Autodesk Inventor part; units mm, degrees
ref_plane "YZ Plane" through (0, 0, 0) normal (1, 0, 0) x (0, 1, 0)
ref_plane "XZ Plane" through (0, 0, 0) normal (0, 1, 0) x (-1, 0, 0)
ref_plane "XY Plane" through (0, 0, 0) normal (0, 0, 1) x (1, 0, 0)
sketch "Sketch1" plane through (0, 0, 0) normal (0, 0, 1) x (1, 0, 0)
  circle A0 centre (8.7376, -2.3876) radius 2.032
  circle A1 centre (-8.7376, -2.3876) radius 2.032
  arc A2 (9.5508, 6.3501) -> (10.564, 6.3532) centre (10.0574, 6.3501) ccw
  line L0 (9.5508, 6.3501) -> (6.3306, 6.3501)
  arc A3 (5.3174, 6.3501) -> (6.3306, 6.3501) centre (5.824, 6.3501) ccw
  line L1 (5.3174, 6.3501) -> (4.2872, 6.3501)
  arc A4 (4.2872, 6.3501) -> (3.2382, 5.3011) centre (4.2872, 5.3011) ccw
  line L2 (3.2382, 5.3011) -> (3.2382, 5.1893)
  arc A5 (3.2382, 5.1893) -> (4.2872, 4.1403) centre (4.2872, 5.1893) ccw
  line L3 (4.2872, 4.1403) -> (6.5409, 4.1403)
  arc A6 (7.2003, 2.5463) -> (6.5409, 4.1403) centre (6.5409, 3.2069) ccw
  line L4 (7.2003, 2.5463) -> (3.8742, -0.7738)
  arc A7 (1.6311, -1.7017) -> (3.8742, -0.7738) centre (1.6311, 1.4733) ccw
  line L5 (1.6311, -1.7017) -> (-1.6318, -1.7017)
  arc A8 (-3.8748, -0.7738) -> (-1.6318, -1.7017) centre (-1.6318, 1.4733) ccw
  line L6 (-3.8748, -0.7738) -> (-7.092, 2.4374)
  arc A9 (-6.3875, 4.1403) -> (-7.092, 2.4374) centre (-6.3875, 3.1432) ccw
  line L7 (-6.3875, 4.1403) -> (-4.2879, 4.1403)
  arc A10 (-4.2879, 4.1403) -> (-3.2388, 5.1893) centre (-4.2879, 5.1893) ccw
  line L8 (-3.2388, 5.1893) -> (-3.2388, 5.3011)
  arc A11 (-3.2388, 5.3011) -> (-4.2879, 6.3501) centre (-4.2879, 5.3011) ccw
  line L9 (-4.2879, 6.3501) -> (-5.3196, 6.3501)
  arc A12 (-6.3328, 6.3501) -> (-5.3196, 6.3501) centre (-5.8262, 6.3501) ccw
  line L10 (-6.3328, 6.3501) -> (-9.5528, 6.3501)
  arc A13 (-10.566, 6.3457) -> (-9.5528, 6.3501) centre (-10.0594, 6.3501) ccw
  line L11 (-10.566, 6.3457) -> (-10.5916, 6.3457)
  arc A14 (-10.5916, 6.3457) -> (-12.7, 4.2373) centre (-10.5916, 4.2373) ccw
  line L12 (-12.7, 4.2373) -> (-12.7, -4.2331)
  arc A15 (-12.7, -4.2331) -> (-10.5647, -6.3413) centre (-10.5916, -4.2331) ccw
  arc A16 (-9.5516, -6.35) -> (-10.5647, -6.3413) centre (-10.0581, -6.3412) ccw
  line L13 (-9.5516, -6.35) -> (-6.323, -6.35)
  arc A17 (-5.31, -6.35) -> (-6.323, -6.35) centre (-5.8165, -6.3412) ccw
  line L14 (-5.31, -6.35) -> (5.31, -6.35)
  arc A18 (6.323, -6.35) -> (5.31, -6.35) centre (5.8165, -6.3412) ccw
  line L15 (6.323, -6.35) -> (9.5502, -6.35)
  arc A19 (10.5633, -6.3403) -> (9.5502, -6.35) centre (10.0567, -6.3412) ccw
  line L16 (10.5633, -6.3403) -> (10.589, -6.3404)
  arc A20 (10.589, -6.3404) -> (12.6991, -4.2321) centre (10.5907, -4.2321) ccw
  line L17 (12.6991, -4.2321) -> (12.6991, 4.2448)
  arc A21 (12.6991, 4.2448) -> (10.5907, 6.3532) centre (10.5907, 4.2448) ccw
  line L18 (10.5907, 6.3532) -> (10.564, 6.3532)
  point P0 (0, 0)
extrude "Extrusion1" add sketch "Sketch1" against normal blind 635
properties part number "25in_1050"
Input: part model. Units: mm. Frame: model coordinates. Coordinates: 2 decimals unless noted, no trailing zeros. Write item = value, one per line. Start each with the question number.
(1) Section A-A on z = -245. Give the number of separate pieces and of enclosed holes in the cut face, and give its area (3 significant figures).
(2) First-contact query: P1, Ø1, axis at x = -8.5, z = -384, coming from the +Y side; P2, Ø5.5, axis at x = -8.74, y = -2.39, coming from the -Z side; P3, Ø3.5, axis at x = 0.5, z = -209, coming from the +Y side. Flat tips, straight axial feed; report the tip coordinate or a pass-through.
(3) Line query: line 1 along X through (y, z) = (-2.5, -561); line 2 along X through (y, z) = (-2, -461); line 3 along X through (y, z) = (6, -125.5). Output: solid intervals per line, ascending. Write a range as [from, to].
Result set:
q1.separate_pieces = 1
q1.enclosed_holes = 2
q1.area = 208 mm²
q2.P1 = 6.35
q2.P2 = -635
q2.P3 = -1.64
q3.line_1 = [-12.7, -10.77], [-6.71, 6.71], [10.77, 12.7]
q3.line_2 = [-12.7, -10.73], [-6.74, 6.74], [10.73, 12.7]
q3.line_3 = [-11.75, -10.43], [-9.69, -6.19], [-5.46, -3.51], [3.5, 5.46], [6.19, 9.69], [10.42, 11.76]
